from build123d import *

# Parameters (mm, degrees)
SKETCH1_W           = 56
SKETCH1_H           = 37.25
BOSS_EXTRUDE1_DEPTH = 2
SKETCH2_W           = 56
SKETCH2_H           = 37.25
SKETCH2_W_2         = 52
SKETCH2_H_2         = 33.25
BOSS_EXTRUDE2_DEPTH = 8.5
SKETCH5_W           = 54
SKETCH5_H           = 35.25
SKETCH5_W_2         = 52
SKETCH5_H_2         = 33.25
CUT_EXTRUDE1_DEPTH  = 1
FILLET1_R           = 1
SKETCH7_W           = 30
SKETCH7_H           = 14
CUT_EXTRUDE3_DEPTH  = 10
SKETCH8_R           = 1.75
CUT_EXTRUDE4_DEPTH  = 10
SKETCH9_W           = 7
SKETCH9_H           = 6
CUT_EXTRUDE5_DEPTH  = 3
SKETCH10_W          = 10
SKETCH10_H          = 2.5
CUT_EXTRUDE6_DEPTH  = 3
FILLET2_R           = 0.5
SKETCH11_W          = 14
SKETCH11_H          = 10
CUT_EXTRUDE7_DEPTH  = 11.5
FILLET3_R           = 1
FILLET4_R           = 0.5
FILLET5_R           = 0.2
CUT_EXTRUDE8_DEPTH  = 0.7


with BuildPart() as part:
    # Sketch1 → Boss-Extrude1 (new body)
    with BuildSketch(Plane(origin=(0, 0, 0), x_dir=(1, 0, 0), z_dir=(0, 1, 0))):
        with Locations((28, 18.625)):
            Rectangle(SKETCH1_W, SKETCH1_H)
    extrude(amount=BOSS_EXTRUDE1_DEPTH)

    # Sketch2 → Boss-Extrude2 (add)
    with BuildSketch(Plane(origin=(0, 2, 0), x_dir=(1, 0, 0), z_dir=(0, 1, 0))):
        with Locations((28, 18.625)):
            Rectangle(SKETCH2_W, SKETCH2_H)
        with Locations((28, 18.625)):
            Rectangle(SKETCH2_W_2, SKETCH2_H_2, mode=Mode.SUBTRACT)
    extrude(amount=BOSS_EXTRUDE2_DEPTH)

    # Sketch5 → Cut-Extrude1 (cut)
    with BuildSketch(Plane(origin=(0, 10.5, 0), x_dir=(1, 0, 0), z_dir=(0, 1, 0))):
        with Locations((28, 18.625)):
            Rectangle(SKETCH5_W, SKETCH5_H)
        with Locations((28, 18.625)):
            Rectangle(SKETCH5_W_2, SKETCH5_H_2, mode=Mode.SUBTRACT)
        with Locations((28, 18.625)):
            Rectangle(SKETCH5_W_2, SKETCH5_H_2)
    extrude(amount=-CUT_EXTRUDE1_DEPTH, mode=Mode.SUBTRACT)

    # Fillet1
    fillet1_edges = [part.edges().sort_by_distance(p)[0] for p in [
        (0, 5.25, -37.25),
        (56, 5.25, -37.25),
        (56, 5.25, 0),
        (0, 5.25, 0),
    ]]
    fillet(fillet1_edges, radius=FILLET1_R)

    # Sketch7 → Cut-Extrude3 (cut)
    with BuildSketch(Plane(origin=(0, 2, 0), x_dir=(1, 0, 0), z_dir=(0, 1, 0))):
        with Locations((31, 13)):
            Rectangle(SKETCH7_W, SKETCH7_H)
    extrude(amount=-CUT_EXTRUDE3_DEPTH, mode=Mode.SUBTRACT)

    # Sketch8 → Cut-Extrude4 (cut)
    with BuildSketch(Plane.XZ):
        with Locations((29.24999924, -23.74999914)):
            Circle(SKETCH8_R)
        with Locations((37.25000102, -23.74999914)):
            Circle(SKETCH8_R)
    extrude(amount=-CUT_EXTRUDE4_DEPTH, mode=Mode.SUBTRACT)

    # Sketch9 → Cut-Extrude5 (cut)
    with BuildSketch(Plane(origin=(0, 0, -37.25), x_dir=(-1, 0, 0), z_dir=(0, 0, -1))):
        with Locations((-47.5, 7.5)):
            Rectangle(SKETCH9_W, SKETCH9_H)
    extrude(amount=-CUT_EXTRUDE5_DEPTH, mode=Mode.SUBTRACT)

    # Sketch10 → Cut-Extrude6 (cut)
    with BuildSketch(Plane(origin=(0, 0, -37.25), x_dir=(-1, 0, 0), z_dir=(0, 0, -1))):
        with Locations((-39, 9.25)):
            Rectangle(SKETCH10_W, SKETCH10_H)
    extrude(amount=-CUT_EXTRUDE6_DEPTH, mode=Mode.SUBTRACT)

    # Fillet2
    fillet2_edges = [part.edges().sort_by_distance(p)[0] for p in [
        (16, 1, -6),
        (16, 1, -20),
        (46, 1, -20),
        (46, 1, -6),
    ]]
    fillet(fillet2_edges, radius=FILLET2_R)

    # Sketch11 → Cut-Extrude7 (cut, through all)
    with BuildSketch(Plane.XZ):
        with Locations((7, -19.2710001)):
            Rectangle(SKETCH11_W, SKETCH11_H)
    extrude(amount=-CUT_EXTRUDE7_DEPTH, mode=Mode.SUBTRACT)

    # Fillet3
    fillet3_edges = [part.edges().sort_by_distance(p)[0] for p in [
        (0, 0, -30.26050005),
        (0.292893219, 0, -0.292893219),
        (28, 0, 0),
        (55.707106781, 0, -0.292893219),
        (56, 0, -18.625),
        (55.707106781, 0, -36.957106781),
        (0.292893219, 0, -36.957106781),
        (28, 0, -37.25),
    ]]
    fillet(fillet3_edges, radius=FILLET3_R)

    # Fillet4
    fillet4_edges = [part.edges().sort_by_distance(p)[0] for p in [
        (14, 1, -24.2710001),
        (14, 1, -14.2710001),
    ]]
    fillet(fillet4_edges, radius=FILLET4_R)

    # Fillet5
    fillet5_edges = [part.edges().sort_by_distance(p)[0] for p in [
        (51, 4.5, -36.25),
        (44, 4.5, -36.25),
        (44, 8, -36.25),
        (34, 8, -36.25),
    ]]
    fillet(fillet5_edges, radius=FILLET5_R)

    # Sketch12 → Cut-Extrude8 (cut)
    with BuildSketch(Plane(origin=(0, 9.5, 0), x_dir=(1, 0, 0), z_dir=(0, 1, 0))):
        Polygon((2, 14.2710001), (1, 14.2710001), (1, 1), (55, 1), (55, 36.25), (51, 36.25), (51, 35.25), (54, 35.25), (54, 2), (2, 2), align=None)
        Polygon((1, 24.2710001), (2, 24.2710001), (2, 35.25), (34, 35.25), (34, 36.25), (1, 36.25), align=None)
    extrude(amount=-CUT_EXTRUDE8_DEPTH, mode=Mode.SUBTRACT)


solid = part.part
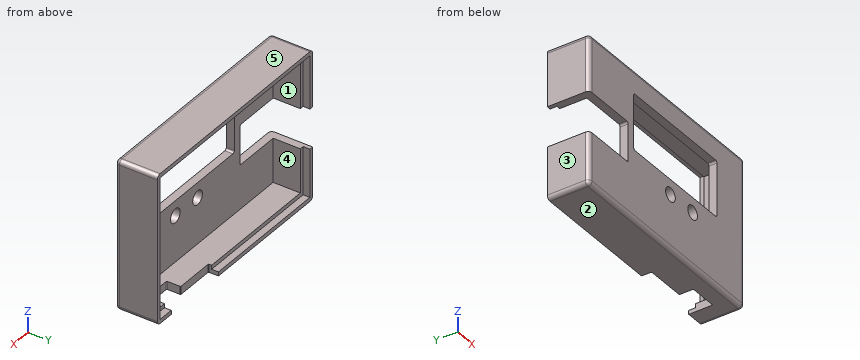
Design review of the part built by this model. Coordinates are the model's own, in mm. Face numbers are marked on the shaded views. A direction names the side the tool comes from. Round coordinates to 2 decimals unless told otherwise and drop trailing zeros. Write each loop counter-clockwise with the first axis right and the second up, starting at its lowest first coordinate (ties: lowest second). Pieces come first, ordered by that corner, then holes. Notation, with made-up numbers: (34, 66.25) - (56, 66.25) arc R18 ccw to (56, 89.25) - close; hole circle Ø5 at (84.5, -2). An arc over 180 degrees is marked (long way). Use a Markdown table: item, result. Add a question column.
1. We need section D-D (z = -27). State the section outline as (x, y) points.
2. Mouldability with a two-part tool opening along Z and no side actions: class the marked faces 1, 2 and 3 as +Z half, -Z half, draft (parallel to the pull), parting line (faces both ways), or undercut.
3. We need section A-A (y = 9.5). State the section outline as (x, z) points.
4. Wall thickness on probe 1 along Z at (x, y) = (29.25, 1.65); probe 2 along Z at (x, y) = (20.5, 4.75); probe 3 along X at (y, z) = (7.5, -2.5): over which ranges is each line inside the solid? List them lowest first.
5. For the marked faces 4 and 5, list the 3-axis set-ups (+Z, -Z, +X, -X, +Y, -Y) from which the entire face can be reached by the end or side of a thin tool; tool diameter is ignored.
6. We need section C-C (x = 19.5). State the section outline as (y, z) points, then the cut area to 3 significant figures.
7. We need section B-B (x = 29.25). State the section outline as (y, z) points, then the cut area to 3 significant figures.
8. Clearance check with flat-ended pins moving along their axes: pin 1 (2 mm diameter, centred on y = 1.5, z = -20, fed in from -X); pin 2 (0.6 mm diameter, centred on y = 0.5, z = -11.5, fed in from -X); pin 3 (2 mm diameter, centred on x = 12.5, z = -14, fed in from +Y). State where each tip first meets the part, or that it passes through.
Output:
| question | item | result |
|---|---|---|
| 1 | outline | (0, 1) arc R1 ccw to (1, 0) - (55, 0) arc R1 ccw to (56, 1) - (56, 10.5) - (55, 10.5) - (55, 8.8) - (54, 8.8) - (54, 2) - (2, 2) - (2, 8.8) - (1, 8.8) - (1, 10.5) - (0, 10.5) - close |
| 2 | face 1 | undercut |
| 2 | face 2 | -Z half |
| 2 | face 3 | draft |
| 3 | outline | (0, -36.25) arc R1 ccw to (1, -37.25) - (34, -37.25) - (34, -36.25) - (1, -36.25) - (1, -24.27) - (0, -24.27) - close; (0, -14.27) - (1, -14.27) - (1, -1) - (55, -1) - (55, -36.25) - (51, -36.25) - (51, -37.25) - (55, -37.25) arc R1 ccw to (56, -36.25) - (56, -1) arc R1 ccw to (55, 0) - (1, 0) arc R1 ccw to (0, -1) - close |
| 4 | probe 1 | z = -37.25 to -25.5, -22 to -20, -6 to 0 |
| 4 | probe 2 | z = -37.25 to -35.25, -2 to 0 |
| 4 | probe 3 | x = 0 to 2, 54 to 56 |
| 5 | face 4 | +Y |
| 5 | face 5 | +Z, +X, -X, +Y, -Y |
| 6 | outline | (0, -36.25) arc R1 ccw to (1, -37.25) - (10.5, -37.25) - (10.5, -36.25) - (8.8, -36.25) - (8.8, -35.25) - (2, -35.25) - (2, -20) - (0, -20) - close; (0, -6) - (2, -6) - (2, -2) - (8.8, -2) - (8.8, -1) - (10.5, -1) - (10.5, 0) - (1, 0) arc R1 ccw to (0, -1) - close |
| 6 | area | 76.7 mm2 |
| 7 | outline | (0, -36.25) arc R1 ccw to (1, -37.25) - (10.5, -37.25) - (10.5, -36.25) - (8.8, -36.25) - (8.8, -35.25) - (2, -35.25) - (2, -25.5) - (0, -25.5) - close; (0, -22) - (2, -22) - (2, -20) - (0, -20) - close; (0, -6) - (2, -6) - (2, -2) - (8.8, -2) - (8.8, -1) - (10.5, -1) - (10.5, 0) - (1, 0) arc R1 ccw to (0, -1) - close |
| 7 | area | 69.7 mm2 |
| 8 | pin 1 | stops at x = 14 |
| 8 | pin 2 | stops at x = 0.02 |
| 8 | pin 3 | stops at y = 2 |
